from build123d import *

# Parameters (mm, degrees)
SKETCH1_W = 2
SKETCH1_H = 8.301435116


with BuildPart() as part:
    # Sketch1 → Revolve1 (revolve)
    with BuildSketch(Plane.XY, mode=Mode.PRIVATE) as revolve1_sk:
        with BuildLine():
            Line((140.585266778, 156.530694973), (139.388010351, 154.928640963))
            ThreePointArc((139.388010351, 154.928640963), (135.261851196, 155.978216625), (131.60205401, 153.802743574))
            ThreePointArc((131.60205401, 153.802743574), (122.652775657, 136.667391705), (119.566449184, 117.583774238))
            ThreePointArc((119.566449184, 117.583774238), (84.552372574, 33.026327641), (0, -2))
            Line((0, -2), (0, 0))
            ThreePointArc((0, 0), (83.138056564, 34.440438748), (117.566449205, 117.583484461))
            ThreePointArc((117.566449205, 117.583484461), (120.754822164, 137.298083815), (130, 155))
            ThreePointArc((130, 155), (134.97561608, 157.957628017), (140.585266778, 156.530694973))
        make_face()
        with Locations((42.774792242, 2.150717558)):
            Rectangle(SKETCH1_W, SKETCH1_H)
    revolve(revolve1_sk.sketch.rotate(Axis((0, 0, 0), (0, -1, 0)), 180), axis=Axis((0, 0, 0), (0, -1, 0)))


solid = part.part
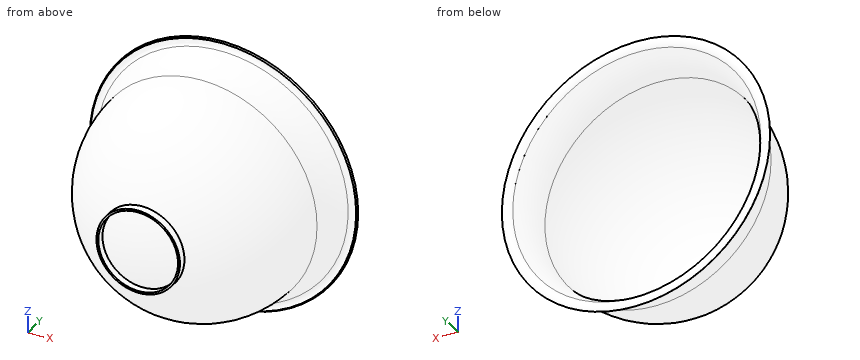
Design review of the part built by this model. Coordinates are the model's own, in mm. Coordinates: 2 decimals unless noted, no trailing zeros. Order: outer loops, then holes, each group sorted by start corner. A loop starts at its lowest first (then second) coordinate and runs counter-clockwise, first axis right, second up. Notation, with made-up numbers: (47, -8) - (83, -8) arc R34 cw to (83, 30) - close; hole circle Ø3 at (-3, 61.5). An arc over 180 degrees is marked (long way). Put each result on its own line as item: value.
1) Take a section at B-B, the plane x = 0. Give the boundary of the cut face in (y, z).
Response values:
outline: (-2, -43.77) - (6.3, -43.77) arc R119.57 ccw to (117.58, -119.57) arc R60.49 cw to (153.8, -131.6) arc R5.56 cw to (154.93, -139.39) - (156.53, -140.59) arc R7.56 ccw to (155, -130) arc R62.49 ccw to (117.58, -117.57) arc R117.57 cw to (117.58, 117.57) arc R62.49 ccw to (155, 130) arc R7.56 ccw to (156.53, 140.59) - (154.93, 139.39) arc R5.56 cw to (153.8, 131.6) arc R60.49 cw to (117.58, 119.57) arc R119.57 ccw to (6.3, 43.77) - (-2, 43.77) - (-2, 41.77) - (5.54, 41.77) arc R119.57 ccw to (5.54, -41.77) - (-2, -41.77) - close
2) Take a section at C-C, the plane y = 128. Give the boundary of the cut face in (x, z).
Response values:
outline: circle Ø240.94 at (0, 0); hole circle Ø236.88 at (0, 0)
3) Insertion check: P1, Ø10, axis at x = -24.5, y = 56, coming from the +Z side; P2, Ø6, axis at x = 33.5, y = 51, coming from the +Z side; P3, Ø10, axis at y = 90, z = 112.5, coming from the -X side. Each pin has a flat end and moves straight along its axis. Give the tip position at first contact, or say it passes through.
Response values:
P1: stops at z = 102.68
P2: stops at z = 95.82
P3: stops at x = -44.87
4) Take a section at A-A, the plane z = 0. Give the boundary of the cut face in (x, y).
Response values:
outline: (-140.59, 156.53) - (-139.39, 154.93) arc R5.56 cw to (-131.6, 153.8) arc R60.49 cw to (-119.57, 117.58) arc R119.57 ccw to (-43.77, 6.3) - (-43.77, -2) - (-41.77, -2) - (-41.77, 5.54) arc R119.57 ccw to (41.77, 5.54) - (41.77, -2) - (43.77, -2) - (43.77, 6.3) arc R119.57 ccw to (119.57, 117.58) arc R60.49 cw to (131.6, 153.8) arc R5.56 cw to (139.39, 154.93) - (140.59, 156.53) arc R7.56 ccw to (130, 155) arc R62.49 ccw to (117.57, 117.58) arc R117.57 cw to (-117.57, 117.58) arc R62.49 ccw to (-130, 155) arc R7.56 ccw to start
5) Take a section at D-D, the plane y = 63. Give the boundary of the cut face in (x, z).
Response values:
outline: circle Ø212.78 at (0, 0); hole circle Ø208.27 at (0, 0)
6) Wall thickness on L1, parallel to Z at x = -60.5, y = 47; L2, parallel to Z at x = 87.5, y = 78; L3, parallel to X at y = 71.5, z = 83: over which ranges is each line inside the solid? List them lowest first. Write a range as from..to.
Response values:
L1: z = -75.21..-71.99, 71.99..75.21
L2: z = -71.23..-67.82, 67.82..71.23
L3: x = -72.7..-69.36, 69.36..72.7
